```python
from build123d import *

# Parameters (mm, degrees)
F1_DEPTH = 320
F2_R     = 5
F3_DEPTH = 1.2
F4_R     = 5
F5_R     = 2.5
F6_DEPTH = 1.2


with BuildPart() as f1:
    # F0 (on Front) → F1 (new body)
    with BuildSketch(Plane.XZ):
        with BuildLine():
            Line((1.2, 0), (0, 0))
            Line((0, 0), (0, -187))
            ThreePointArc((0, -187), (-1.464466, -190.535534), (-5, -192))
            Line((-5, -192), (-30, -192))
            Line((-30, -192), (-30, -193.2))
            Line((-30, -193.2), (-5, -193.2))
            ThreePointArc((-5, -193.2), (-0.615938, -191.384062), (1.2, -187))
            Line((1.2, -187), (1.2, 0))
        make_face()
    extrude(amount=-F1_DEPTH)

    # F2 (on face) → F3 (cut, through all)
    with BuildSketch(Plane.XY.offset(-192)):
        with Locations((-17.5, 305)):
            Circle(F2_R)
        with Locations((-17.5, 15)):
            Circle(F2_R)
    extrude(amount=-F3_DEPTH, mode=Mode.SUBTRACT)

    # F4
    f4_edges = [f1.edges().sort_by_distance(p)[0] for p in [
        (-30, 320, -192.6),
        (-30, 0, -192.6),
    ]]
    fillet(f4_edges, radius=F4_R)

    # F5 (on face) → F6 (cut, through all)
    with BuildSketch(Plane.YZ.offset(1.2)):
        with Locations((10, -20)):
            Circle(F5_R)
        with Locations((160, -20)):
            Circle(F5_R)
        with Locations((310, -20)):
            Circle(F5_R)
    extrude(amount=-F6_DEPTH, mode=Mode.SUBTRACT)


solid = f1.part
```
CAD build for the part. Positions are in the model's coordinates, mm. Coordinates: 2 decimals unless noted, no trailing zeros. Order: outer loops, then holes, each group sorted by start corner. A loop starts at its lowest first (then second) coordinate and runs counter-clockwise, first axis right, second up. Notation, with made-up numbers: (29.5, 37) - (62.5, 37) arc R26 ccw to (62.5, 68) - close; hole circle Ø11 at (30.5, 4.5). An arc over 180 degrees is marked (long way). Answer in a Markdown table with one row per item.
1. Slice it at A-A, the plane x = -17.5. List the corners of the cut face in (y, z).
Answer:
| item | result |
|---|---|
| outline | (0, -193.2) - (10, -193.2) - (10, -192) - (0, -192) - close; (20, -193.2) - (300, -193.2) - (300, -192) - (20, -192) - close; (310, -193.2) - (320, -193.2) - (320, -192) - (310, -192) - close |
2. Slice it at C-C, the plane z = -35.5. List the corners of the cut face in (x, y).
Answer:
| item | result |
|---|---|
| outline | (0, 0) - (1.2, 0) - (1.2, 320) - (0, 320) - close |
3. Drill centre lines: L1, parallel to Y at x = -17.5, z = -192.6; L2, parallel to Z at x = -13, y = 32; L3, parallel to X at y = 181.5, z = -27.5. Where is each one in solid material? Low to high. Write a range as from..to.
Answer:
| item | result |
|---|---|
| L1 | 0..10, 20..300, 310..320 |
| L2 | -193.2..-192 |
| L3 | 0..1.2 |
4. Flat gauge pins, fed straight in: P1, Ø1, axis at x = -10, y = 103, coming from the +Z side; P2, Ø6.5, axis at y = 10, z = -20, coming from the -X side. Where does each tip first touch, or does it go through?
Answer:
| item | result |
|---|---|
| P1 | z = -192 |
| P2 | x = 0 |
5. Pull direction X, two halves, no side cores. Call faces 1 (the face through (-17, 158, -192)), 2 (the face through (-18.58, 10.12, -192.59)), 3 (the face through (0, 158, -92)): +X half, -X half, draft (parallel to the pull), parting line (faces both ways), or undercut.
Answer:
| item | result |
|---|---|
| face 1 | draft |
| face 2 | undercut |
| face 3 | -X half |
6. Slice it at B-B, the plane y = 242. List the corners of the cut face in (x, z), then the cut area to 3 significant figures.
Answer:
| item | result |
|---|---|
| outline | (-30, -193.2) - (-5, -193.2) arc R6.2 ccw to (1.2, -187) - (1.2, 0) - (0, 0) - (0, -187) arc R5 cw to (-5, -192) - (-30, -192) - close |
| area | 265 mm² |
